from build123d import *

# Parameters (mm, degrees)
SKETCH_1_R                   = 18
SKETCH_1_R_2                 = 1.1
SKETCH_1_R_3                 = 1.6
EXTRUDE_1_DEPTH              = 7
SKETCH_5_R                   = 2.1
CUT_EXTRUDE_1_DEPTH          = 5.6
HOLE_WIZARD_M3_2_D           = 3.6
HOLE_WIZARD_M3_2_CSINK_D     = 6.3
HOLE_WIZARD_M3_2_CSINK_ANGLE = 90


with BuildPart() as part:
    # 스케치1 → 보스-돌출1 (new body)
    with BuildSketch(Plane.XY):
        Circle(SKETCH_1_R)
        with Locations((0, 4)):
            Circle(SKETCH_1_R_2, mode=Mode.SUBTRACT)
        with Locations((4, 0)):
            Circle(SKETCH_1_R_2, mode=Mode.SUBTRACT)
        with Locations((0, -4)):
            Circle(SKETCH_1_R_2, mode=Mode.SUBTRACT)
        with Locations((-4, 0)):
            Circle(SKETCH_1_R_2, mode=Mode.SUBTRACT)
        with Locations((-13.249665953, 4.822484021)):
            Circle(SKETCH_1_R_3, mode=Mode.SUBTRACT)
        with Locations((-13.249665953, -4.822484021)):
            Circle(SKETCH_1_R_3, mode=Mode.SUBTRACT)
        with Locations((10.801226648, 9.063305297)):
            Circle(SKETCH_1_R_3, mode=Mode.SUBTRACT)
        with Locations((2.448439305, 13.885789317)):
            Circle(SKETCH_1_R_3, mode=Mode.SUBTRACT)
        with Locations((2.448439305, -13.885789317)):
            Circle(SKETCH_1_R_3, mode=Mode.SUBTRACT)
        with Locations((10.801226648, -9.063305297)):
            Circle(SKETCH_1_R_3, mode=Mode.SUBTRACT)
    extrude(amount=EXTRUDE_1_DEPTH)

    # 스케치5 → 컷-돌출1 (cut)
    with BuildSketch(Plane.XY.offset(7)):
        with Locations((0, 4)):
            Circle(SKETCH_5_R)
        with Locations((0, -4)):
            Circle(SKETCH_5_R)
        with Locations((4, 0)):
            Circle(SKETCH_5_R)
        with Locations((-4, 0)):
            Circle(SKETCH_5_R)
    extrude(amount=-CUT_EXTRUDE_1_DEPTH, mode=Mode.SUBTRACT)

    # M3 접시 머리 나사용 카운터싱크2 (through all)
    with Locations(Plane(origin=(0, 0, 0), x_dir=(-1, 0, 0), z_dir=(0, 0, -1))):
        with Locations((-2.448439305, 13.885789317), (13.249665953, 4.822484021), (13.249665953, -4.822484021), (-2.448439305, -13.885789317), (-10.801226648, -9.063305297), (-10.801226648, 9.063305297)):
            CounterSinkHole(HOLE_WIZARD_M3_2_D / 2, HOLE_WIZARD_M3_2_CSINK_D / 2, counter_sink_angle=HOLE_WIZARD_M3_2_CSINK_ANGLE)


solid = part.part
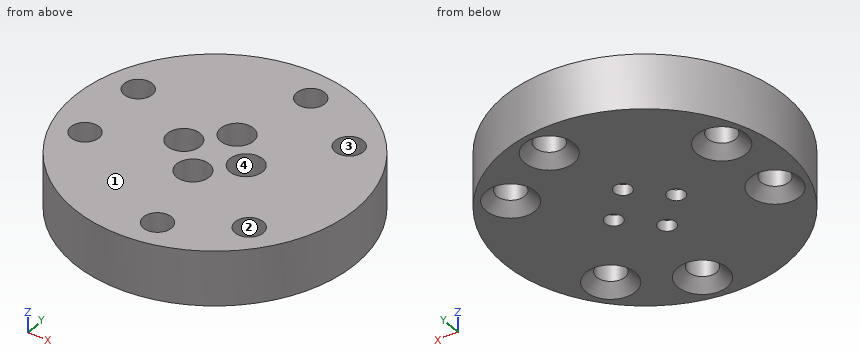
Model file for the job. Use its own axes, mm. Face numbers are marked on the shaded views. A direction names the side the tool comes from. Round coordinates to 2 decimals unless told otherwise and drop trailing zeros. Order: outer loops, then holes, each group sorted by start corner. A loop starts at its lowest first (then second) coordinate and runs counter-clockwise, first axis right, second up.
(1) Drill centre lines: line 1 (Y direction, x = 0, z = 0.75); line 2 (Y direction, x = -1, z = 5.75); line 3 (Y direction, x = 4, z = 3). Where is each one in solid material? Low to high.
(2) Band-saw the part on C-C (z = 4.5). Give the number of separate pieces and of enclosed holes in the cut face, then the cut area to 3 significant figures.
(3) Band-saw the part on A-A (y = 0). List the corners of the cut face in (x, z), then the cut area to 3 significant figures.
(4) Band-saw the part on B-B (x = -4). List the corners of the cut face in (y, z).
(5) Pull direction X, two halves, no side cores. Call the marked faces 1 and 2: released by +X, released by -X, zero draft, split by the parting line, or undercut.
(6) Pin check, flat tips, straight feed: pin 1 (1.3 mm diameter, centred on x = 0, y = -3, fed in from +Z); pin 2 (2 mm diameter, centred on y = 9, z = 6, fed in from -X); pin 3 (3 mm diameter, centred on y = -11.5, z = 1, fed in from +X); pin 4 (1.3 mm diameter, centred on x = 0, y = -4, fed in from -Z). Stop position of each tip, or through.
(7) 3-axis set-ups, long thin cutter, end or side, ignore diameter. For the marked faces 3 and 4: which of +Z, -Z, +X, -X, +Y, -Y reach the whole face in a straight line?
Verdict:
1. line 1: y = -18 to -5.1, -2.9 to 2.9, 5.1 to 18
1. line 2: y = -17.97 to -5.85, -2.15 to 2.15, 5.85 to 17.97
1. line 3: y = -17.55 to -14.8, -12.97 to -2.1, 2.1 to 12.97, 14.8 to 17.55
2. separate pieces: 1
2. enclosed holes: 10
2. area: 901 mm2
3. outline: (-18, 0) - (-5.1, 0) - (-5.1, 1.4) - (-6.1, 1.4) - (-6.1, 7) - (-18, 7) - close; (-2.9, 0) - (2.9, 0) - (2.9, 1.4) - (1.9, 1.4) - (1.9, 7) - (-1.9, 7) - (-1.9, 1.4) - (-2.9, 1.4) - close; (5.1, 0) - (18, 0) - (18, 7) - (6.1, 7) - (6.1, 1.4) - (5.1, 1.4) - close
3. area: 199 mm2
4. outline: (-17.55, 0) - (-1.1, 0) - (-1.1, 1.4) - (-2.1, 1.4) - (-2.1, 7) - (-17.55, 7) - close; (1.1, 0) - (17.55, 0) - (17.55, 7) - (2.1, 7) - (2.1, 1.4) - (1.1, 1.4) - close
5. face 1: zero draft
5. face 2: undercut
6. pin 1: stops at z = 1.4
6. pin 2: stops at x = -16.12
6. pin 3: stops at x = 14.97
6. pin 4: passes through
7. face 3: +Z, -Z
7. face 4: +Z
